Work out the finished part from the listing and answer in its coordinate system (mm). Face numbers are marked on the shaded views. A direction names the side the tool comes from. Give positions to 0.01 mm unless a question says otherwise; leave off trailing zeros. Order: outer loops, then holes, each group sorted by start corner. A loop starts at its lowest first (then second) coordinate and runs counter-clockwise, first axis right, second up. Notation, with made-up numbers: (-38.5, -15) -> (-2.5, -15) arc R10 cw to (-2.5, 0) -> close; hole circle Ø8 at (78, -15.75). An arc over 180 degrees is marked (long way). Answer as CSV lines item,"result". Start each with the question number.
1. A cutting plane is placed at C-C (y = -11.25). Give the vertices of the cut face in (x, z).
2. For the marked faces 1 and 2, determine the directions among +Z, -Z, +X, -X, +Y, -Y from which every point of the face is accessible in a straight line to the end or side of a thin tool.
3. A cutting plane is placed at B-B (z = 0). Give the vertices of the cut face in (x, y), then the cut area to 3 significant figures.
4. Find the intervals of material crossed by L1, parallel to Z at x = 0, y = -21.75; L2, parallel to Z at x = 0, y = -9.25; L3, parallel to Z at x = 0, y = -12.5, in increasing order.
5. A cutting plane is placed at D-D (x = -7.5). Give the vertices of the cut face in (y, z), then the cut area to 3 significant figures.
6. For a pull along Z with two mould halves and no side action, classify the marked faces 3, 4 and 5 as released by +Z, released by -Z, zero draft, split by the parting line, or undercut.
7. Flat-ended cylindrical pins translate along their axes: pin 1 (5 mm diameter, centred on x = 21.5, z = 2, fed in from +Y); pin 2 (6 mm diameter, centred on x = 16.5, y = -16.5, fed in from -Z); pin 3 (10 mm diameter, centred on y = -20, z = -12, fed in from -X); pin 4 (10 mm diameter, centred on x = 24, z = -12, fed in from -Y). Find the tip coordinate at first contact, or state that the pin passes through.
8. A cutting plane is placed at A-A (x = 0). Give the vertices of the cut face in (y, z), then the cut area to 3 significant figures.
from build123d import *

# Parameters (mm, degrees)
ESQUISSE4_R           = 1.5
EXTRUSION3_DEPTH      = 25
ESQUISSE5_OUTSIDE_W   = 153.718
ESQUISSE5_OUTSIDE_H   = 153.718
ESQUISSE5_OUTSIDE_W_2 = 71
ESQUISSE5_OUTSIDE_H_2 = 48
EXTRUSION4_DEPTH      = 13


with BuildPart() as part:
    # Esquisse1 → Révolution1 (revolve)
    with BuildSketch(Plane.XY):
        Polygon((19, -12), (59, -12), (59, 0), (15, 0), (15, -20), (9, -20), (9, -24), (19, -24), align=None)
    revolve(axis=Axis((0, 0, 0), (0, -1, 0)))

    # Esquisse4 → Extrusion3 (cut, through all)
    with BuildSketch(Plane.XZ.offset(24)):
        with Locations((0, 13)):
            Circle(ESQUISSE4_R)
        with Locations((13, 0)):
            Circle(ESQUISSE4_R)
        with Locations((0, -13)):
            Circle(ESQUISSE4_R)
        with Locations((-13, 0)):
            Circle(ESQUISSE4_R)
    extrude(amount=-EXTRUSION3_DEPTH, mode=Mode.SUBTRACT)

    # Esquisse5 outside → Extrusion4 (cut, through all)
    with BuildSketch(Plane.XZ.offset(12)):
        Rectangle(ESQUISSE5_OUTSIDE_W, ESQUISSE5_OUTSIDE_H)
        Rectangle(ESQUISSE5_OUTSIDE_W_2, ESQUISSE5_OUTSIDE_H_2, mode=Mode.SUBTRACT)
    extrude(amount=-EXTRUSION4_DEPTH, mode=Mode.SUBTRACT)


solid = part.part
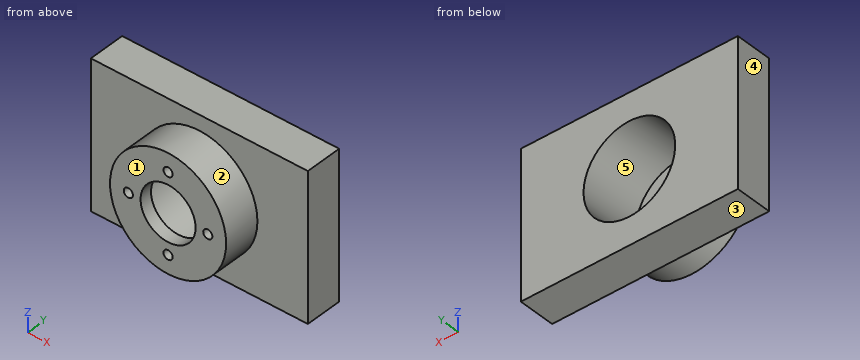
Answer sheet:
1,outline,"(-35.5, -24) -> (35.5, -24) -> (35.5, 24) -> (-35.5, 24) -> close; hole circle Ø30 at (0, 0)"
2,face 1,"+Z, -Z, +X, -X, -Y"
2,face 2,"-Y"
3,outline,"(-35.5, -12) -> (-19, -12) -> (-19, -24) -> (-14.5, -24) -> (-14.5, -20) -> (-15, -20) -> (-15, 0) -> (-35.5, 0) -> close; (-11.5, -24) -> (-9, -24) -> (-9, -20) -> (-11.5, -20) -> close; (9, -24) -> (11.5, -24) -> (11.5, -20) -> (9, -20) -> close; (14.5, -24) -> (19, -24) -> (19, -12) -> (35.5, -12) -> (35.5, 0) -> (15, 0) -> (15, -20) -> (14.5, -20) -> close"
3,area,"612 mm^2"
4,L1,"z = -19 to -14.5, -11.5 to -9, 9 to 11.5, 14.5 to 19"
4,L2,"z = -24 to -15, 15 to 24"
4,L3,"z = -19 to -15, 15 to 19"
5,outline,"(-24, -17.46) -> (-12, -17.46) -> (-12, -24) -> (0, -24) -> (0, -12.99) -> (-20, -12.99) -> (-20, -4.97) -> (-24, -4.97) -> close; (-24, 4.97) -> (-20, 4.97) -> (-20, 12.99) -> (0, 12.99) -> (0, 24) -> (-12, 24) -> (-12, 17.46) -> (-24, 17.46) -> close"
5,area,"436 mm^2"
6,face 3,"released by -Z"
6,face 4,"zero draft"
6,face 5,"undercut"
7,pin 1,"stops at y = 0"
7,pin 2,"stops at z = -13.37"
7,pin 3,"stops at x = -17.66"
7,pin 4,"stops at y = -12"
8,outline,"(-24, -19) -> (-12, -19) -> (-12, -24) -> (0, -24) -> (0, -15) -> (-20, -15) -> (-20, -14.5) -> (-24, -14.5) -> close; (-24, -11.5) -> (-20, -11.5) -> (-20, -9) -> (-24, -9) -> close; (-24, 9) -> (-20, 9) -> (-20, 11.5) -> (-24, 11.5) -> close; (-24, 14.5) -> (-20, 14.5) -> (-20, 15) -> (0, 15) -> (0, 24) -> (-12, 24) -> (-12, 19) -> (-24, 19) -> close"
8,area,"336 mm^2"
